```python
from build123d import *

# Parameters (mm, degrees)
F0_W     = 30
F0_H     = 30
F1_DEPTH = 2
F0_W_2   = 2
F0_H_2   = 1.9999989867
F0_W_3   = 1.9999989867
F0_H_3   = 2
F2_DEPTH = 52


with BuildPart() as f1:
    # F0 (on Top) → F1 (new body)
    with BuildSketch(Plane.XY):
        Polygon((-11.9309425354, 30.1818712056), (-29.8587139696, 30.1818712056), (-29.8587139696, 12.2573869303), (-29.8587139696, 7.1818712056), (-29.8587139696, 5.1818712056), (-29.8587139696, 0.1818712056), (0.1412860304, 0.1818712056), (0.1412860304, 30.1818712056), (-4.8587139696, 30.1818712056), (-4.9099967368, 30.1818712056), (-6.9099967368, 30.1818712056), align=None)
        Polygon((0.1412860304, 0.1818712056), (-29.8587139696, 0.1818712056), (-29.8587139696, -29.8181287944), (-29.847416997, -29.8181287944), (0.1412860304, -29.8181287944), align=None)
        Polygon((30.0900032632, 30.1818712056), (0.1412860304, 30.1818712056), (0.1412860304, 0.1818712056), (30.1412860304, 0.1818712056), (30.1412860304, 30.1818712056), align=None)
        with Locations((15.1412860304, -14.8181287944)):
            Rectangle(F0_W, F0_H)
    extrude(amount=F1_DEPTH)

    # F0 (on Top) → F2 (join)
    with BuildSketch(Plane.XY):
        Polygon((-31.8587129563, 5.1818712056), (-31.8587129563, 7.1818712056), (-35.347416997, 7.1818712056), (-35.347416997, -29.8181287944), (-33.347416997, -29.8181287944), (-33.347416997, 5.1818712056), align=None)
        with Locations((-5.9099967368, 31.1818706989)):
            Rectangle(F0_W_2, F0_H_2)
        Polygon((-6.9099967368, 35.6818712056), (-10.1051449882, 32.1818701923), (-6.9099967368, 32.1818701923), align=None)
        Polygon((-31.8587129563, 7.1818712056), (-31.8587129563, 10.4079470433), (-35.347416997, 7.1818712056), align=None)
        Polygon((-10.1051449882, 32.1818701923), (-11.9309425354, 30.1818712056), (-6.9099967368, 30.1818712056), (-6.9099967368, 32.1818701923), align=None)
        Polygon((-6.9099967368, 35.6818712056), (-6.9099967368, 32.1818701923), (-4.9099967368, 32.1818701923), (-4.9099967368, 33.6818712056), (30.0900032632, 33.6818712056), (30.0900032632, 35.6818712056), align=None)
        Polygon((-29.8587139696, 12.2573869303), (-29.8587139696, 30.1818712056), (-11.9309425354, 30.1818712056), (-10.1051449882, 32.1818701923), (-31.8587129563, 32.1818701923), (-31.8587129563, 10.4079470433), align=None)
        Polygon((-29.8587139696, 7.1818712056), (-29.8587139696, 12.2573869303), (-31.8587129563, 10.4079470433), (-31.8587129563, 7.1818712056), align=None)
        with Locations((-30.8587134629, 6.1818712056)):
            Rectangle(F0_W_3, F0_H_3)
    extrude(amount=F2_DEPTH)


solid = f1.part
```
Can you work these out from the model? Positions are in its coordinate system, mm. A direction names the side the tool comes from. Coordinates: 2 decimals unless noted, no trailing zeros. Loops run counter-clockwise (first coordinate to the right, second up) from the corner with the lowest first, then second, coordinate; pieces in that order, holes last. Notation, with made-up numbers: (-12, 59.25) - (18, 59.25) arc R21 cw to (18, 64.25) - close; hole circle Ø2 at (36, 29.5). An arc over 180 degrees is marked (long way). Answer as CSV lines item,"result". Start each with the question number.
1) I need wall thicknesses on line 1 (Y direction, x = -26.5, z = 10.5); line 2 (X direction, y = 16.5, z = 25); line 3 (X direction, y = 5, z = 46). Which ranges of each line are inside material? Lowest first, please. Write a range as from..to.
2) Suppose I cut it at B-B (x = -2.5). Please give me the cut outline in (y, z).
3) Thinking about a two-plate mould opening in Y: for faces 4 (the flat face through (13, 30.182, 1)), 5 (the flat face through (-29.859, -12, 1)), 6 (the flat face through (-33.6, 8.8, 25.6)), which applies, pulls with the +Y half, pulls with the -Y half, needs draft (parallel to the pull), parting line crosses it, or undercut?
4) For pin 1 (18.5 mm diameter, centred on x = -16, z = 16.5, fed in from -Y); pin 2 (10.5 mm diameter, centred on x = 21, z = 34.5, fed in from -Y); pin 3 (2 mm diameter, centred on x = -15.5, y = -0.5, fed in from +Z), each with a flat end and sliding along its axis, tell me the tip position at first contact or that it passes through.
5) Suppose I cut it at C-C (z = 27). Please give me the cut outline in (x, y).
6) Suppose I cut it at A-A (y = -0.5). Please give me the cut outline in (x, z).
7) Which directions (+Z, -Z, +X, -X, +Y, -Y) give clear straight access to the entire face, cutting with the end or side of a thin tool? Please do faces 1 (the flat face through (-29.859, 18, 27)), 2 (the flat face through (30.09, 35, 26)), 3 (the flat face through (-21, 32.182, 26)).
8) Suppose I cut it at D-D (y = 25.5). Please give me the cut outline in (x, z).
Check result:
1,line 1,"y = 30.18..32.18"
1,line 2,"x = -31.86..-29.86"
1,line 3,"x = -35.35..-33.35"
2,outline,"(-29.82, 0) - (30.18, 0) - (30.18, 2) - (-29.82, 2) - close; (33.68, 0) - (35.68, 0) - (35.68, 52) - (33.68, 52) - close"
3,face 4,"undercut"
3,face 5,"needs draft"
3,face 6,"pulls with the +Y half"
4,pin 1,"stops at y = 30.18"
4,pin 2,"stops at y = 33.68"
4,pin 3,"stops at z = 2"
5,outline,"(-35.35, -29.82) - (-33.35, -29.82) - (-33.35, 5.18) - (-29.86, 5.18) - (-29.86, 30.18) - (-4.91, 30.18) - (-4.91, 33.68) - (30.09, 33.68) - (30.09, 35.68) - (-6.91, 35.68) - (-10.11, 32.18) - (-31.86, 32.18) - (-31.86, 10.41) - (-35.35, 7.18) - close"
6,outline,"(-35.35, 0) - (-33.35, 0) - (-33.35, 52) - (-35.35, 52) - close; (-29.86, 0) - (30.14, 0) - (30.14, 2) - (-29.86, 2) - close"
7,face 1,"+Z, +X, -Y"
7,face 2,"+Z, -Z, +X, +Y, -Y"
7,face 3,"+Z, -Z, -X, +Y"
8,outline,"(-31.86, 0) - (30.14, 0) - (30.14, 2) - (-29.86, 2) - (-29.86, 52) - (-31.86, 52) - close"
